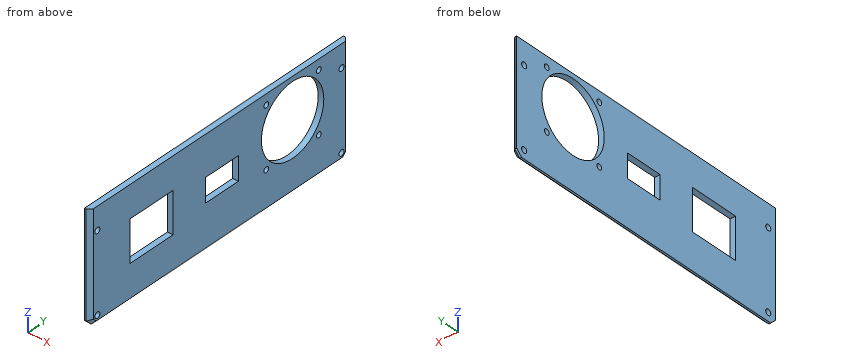
from build123d import *

# Parameters (mm, degrees)
SKETCH012_R     = 1.55
PAD006_DEPTH    = 3
SKETCH013_R     = 1.45
SKETCH013_W     = 26.3
SKETCH013_H     = 22
SKETCH013_W_2   = 20
SKETCH013_H_2   = 12.7
POCKET006_DEPTH = 5
SKETCH014_R     = 19
POCKET007_DEPTH = 5
CHAMFER004_SIZE = 2


with BuildPart() as part:
    # Sketch012 (on ShapeBinder) → Pad006 (new body)
    with BuildSketch(Plane.YZ.offset(280)):
        Polygon((-6.3, -9.3), (-3.3, -12.3), (148.3, -12.3), (151.3, -9.3), (151.3, 46), (-6.3, 46), align=None)
        with Locations((-1.8, 34)):
            Circle(SKETCH012_R, mode=Mode.SUBTRACT)
        with Locations((-1.8, -7.8)):
            Circle(SKETCH012_R, mode=Mode.SUBTRACT)
        with Locations((146.8, -7.8)):
            Circle(SKETCH012_R, mode=Mode.SUBTRACT)
        with Locations((146.8, 34)):
            Circle(SKETCH012_R, mode=Mode.SUBTRACT)
    extrude(amount=PAD006_DEPTH)

    # Sketch013 (on ShapeBinder) → Pocket006 (cut)
    with BuildSketch(Plane.YZ.offset(280)):
        with Locations((101, 40.5)):
            Circle(SKETCH013_R)
        with Locations((133, 40.5)):
            Circle(SKETCH013_R)
        with Locations((101, 8.5)):
            Circle(SKETCH013_R)
        with Locations((133, 8.5)):
            Circle(SKETCH013_R)
        with Locations((31.15, 18)):
            Rectangle(SKETCH013_W, SKETCH013_H)
        with Locations((74, 18.35)):
            Rectangle(SKETCH013_W_2, SKETCH013_H_2)
    extrude(amount=POCKET006_DEPTH, mode=Mode.SUBTRACT)

    # Sketch014 (on Face5 of Pocket006) → Pocket007 (cut)
    with BuildSketch(Plane.YZ.offset(283)):
        with Locations((117, 24.5)):
            Circle(SKETCH014_R)
    extrude(amount=-POCKET007_DEPTH, mode=Mode.SUBTRACT)

    # Chamfer004
    chamfer004_edges = [part.edges().sort_by_distance(p)[0] for p in [
        (283, -6.3, 18.35),
        (283, -4.8, -10.8),
        (283, 72.5, -12.3),
        (283, 149.8, -10.8),
        (283, 151.3, 18.35),
    ]]
    chamfer(chamfer004_edges, length=CHAMFER004_SIZE)


solid = part.part
Geometry check sheet. Reference: the model listing, model coordinates, mm. Give positions to 0.01 mm unless a question says otherwise; leave off trailing zeros. Order: outer loops, then holes, each group sorted by start corner. A loop starts at its lowest first (then second) coordinate and runs counter-clockwise, first axis right, second up.
1) Gauge pin test, flat ends, axial feed: pin 1 (1 mm diameter, centred on x = 282.5, y = 74, fed in from -Z); pin 2 (0.9 mm diameter, centred on x = 281.5, z = 17, fed in from +Y); pin 3 (1 mm diameter, centred on x = 282, z = 30, fed in from +Y). Record the tip position at first contact, or that the pin passes through.
Results are:
pin 1: stops at z = -11.3
pin 2: stops at y = 151.25
pin 3: stops at y = 150.8
2) Cross-section at C-C (y = 101). Record the boundary of the cut face in (x, z).
Results are:
outline: (280, -12.3) - (281, -12.3) - (283, -10.3) - (283, 7.05) - (280, 7.05) - close; (280, 9.95) - (283, 9.95) - (283, 14.25) - (280, 14.25) - close; (280, 34.75) - (283, 34.75) - (283, 39.05) - (280, 39.05) - close; (280, 41.95) - (283, 41.95) - (283, 46) - (280, 46) - close
3) Material ranges on probe 1 along Y at (x, z) = (280.55, 25); probe 2 along Z at (x, y) = (281, -1.8); probe 3 along Y at (x, z) = (280.35, 19.5), recorded low to high.
Results are:
probe 1: y = -6.3 to 18, 44.3 to 98.01, 135.99 to 151.3
probe 2: z = -12.3 to -9.35, -6.25 to 32.45, 35.55 to 46
probe 3: y = -6.3 to 18, 44.3 to 64, 84 to 98.67, 135.33 to 151.3
4) Cross-section at A-A (y = 72). Record the boundary of the cut face in (x, z), then the cut area to 3 significant figures.
Results are:
outline: (280, -12.3) - (281, -12.3) - (283, -10.3) - (283, 12) - (280, 12) - close; (280, 24.7) - (283, 24.7) - (283, 46) - (280, 46) - close
area: 135 mm2
5) Cross-section at D-D (y = 117). Record the boundary of the cut face in (x, z).
Results are:
outline: (280, -12.3) - (281, -12.3) - (283, -10.3) - (283, 5.5) - (280, 5.5) - close; (280, 43.5) - (283, 43.5) - (283, 46) - (280, 46) - close
6) Cross-section at B-B (x = 282.35). Give the number of separate pieces and of enclosed holes in the cut face, then the cut area to 3 significant figures.
Results are:
separate pieces: 1
enclosed holes: 11
area: 6,790 mm2
